Work out the finished part from the listing and answer in its coordinate system (mm). Face numbers are marked on the shaded views. A direction names the side the tool comes from. Coordinates: 2 decimals unless noted, no trailing zeros. Order: outer loops, then holes, each group sorted by start corner. A loop starts at its lowest first (then second) coordinate and runs counter-clockwise, first axis right, second up. Notation, with made-up numbers: M 11,-10.75 L 49,-10.75 A20 ccw 49,-6.75 Z; hole C 51,21 d5. An arc over 180 degrees is marked long. Use a Markdown table: item, result.
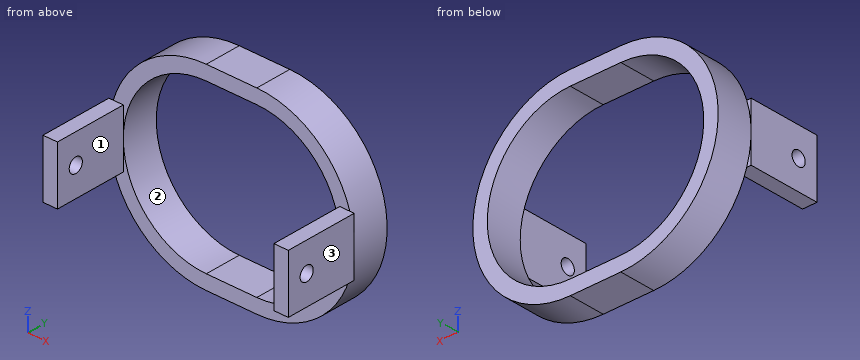
from build123d import *

# Parameters (mm, degrees)
EXTRUDE_1_DEPTH     = 10
SKETCH_3_W          = 4
SKETCH_3_H          = 16
EXTRUDE_2_DEPTH     = 20
SKETCH_5_R          = 2
CUT_EXTRUDE_2_DEPTH = 69


with BuildPart() as part:
    # 草图2 → 凸台-拉伸1 (new body)
    with BuildSketch(Plane(origin=(0, 0, 0), x_dir=(1, 0, 0), z_dir=(0, 1, 0))):
        with BuildLine():
            Line((-7, 27), (7, 27))
            ThreePointArc((7, 27), (34, 0), (7, -27))
            Line((7, -27), (-7, -27))
            ThreePointArc((-7, -27), (-34, 0), (-7, 27))
        make_face()
        with BuildLine():
            Line((-7, 23), (7, 23))
            ThreePointArc((7, 23), (30, 0), (7, -23))
            Line((7, -23), (-7, -23))
            ThreePointArc((-7, -23), (-30, 0), (-7, 23))
        make_face(mode=Mode.SUBTRACT)
    extrude(amount=EXTRUDE_1_DEPTH)

    # 草图3 → 凸台-拉伸2 (add)
    with BuildSketch(Plane.XZ):
        with Locations((-32, 0)):
            Rectangle(SKETCH_3_W, SKETCH_3_H)
        with Locations((32, 0)):
            Rectangle(SKETCH_3_W, SKETCH_3_H)
    extrude(amount=EXTRUDE_2_DEPTH)

    # 草图5 → 切除-拉伸2 (cut, through all)
    with BuildSketch(Plane(origin=(34, 0, 0), x_dir=(0, 0, -1), z_dir=(1, 0, 0))):
        with Locations((0, -14.426533044)):
            Circle(SKETCH_5_R)
    extrude(amount=-CUT_EXTRUDE_2_DEPTH, mode=Mode.SUBTRACT)


solid = part.part
(1) Given P1, Ø1.2, axis at x = 31, y = -14, coming from the +Z side; P2, Ø1.2, axis at x = -31.5, y = -7, coming from the -Z side; P3, Ø12, axis at x = -25, y = 6.5, coming from the -Z side, each flat-ended and moving along its own axis, determine where each tip first touches the part or whether it passes through.
Conclusion:
| item | result |
|---|---|
| P1 | z = 8 |
| P2 | z = -8 |
| P3 | z = -24.19 |
(2) A cutting plane is placed at C-C (x = 14). Determine the outline of the cut face in (y, z).
Conclusion:
| item | result |
|---|---|
| outline | M 0,-26.08 L 10,-26.08 L 10,-21.91 L 0,-21.91 Z; M 0,21.91 L 10,21.91 L 10,26.08 L 0,26.08 Z |
(3) Straight lines are drawn through the part: L1, parallel to Z at x = -4.5, y = 8.5; L2, parallel to Y at x = -32.85, z = 0; L3, parallel to X at y = -17.5, z = -3. For each, find the intervals that lie inside material, in ascending order.
Conclusion:
| item | result |
|---|---|
| L1 | -27 to -23, 23 to 27 |
| L2 | -20 to -16.43, -12.43 to 10 |
| L3 | -34 to -30, 30 to 34 |
(4) A cutting plane is placed at A-A (z = 4). Determine the outline of the cut face in (x, y), then the cut area to 3 significant figures.
Conclusion:
| item | result |
|---|---|
| outline | M -34,-20 L -30,-20 L -30,0 L -29.65,0 L -29.65,10 L -33.7,10 L -33.7,0 L -34,0 Z; M 29.65,0 L 30,0 L 30,-20 L 34,-20 L 34,0 L 33.7,0 L 33.7,10 L 29.65,10 Z |
| area | 241 mm2 |
(5) A cutting plane is placed at D-D (y = 1.25). Determine the outline of the cut face in (x, z), then the cut area to 3 significant figures.
Conclusion:
| item | result |
|---|---|
| outline | M -7,-27 L 7,-27 A27 ccw 7,27 L -7,27 A27 ccw Z; hole M -7,-23 L 7,-23 A23 ccw 7,23 L -7,23 A23 ccw Z |
| area | 740 mm2 |
(6) A cutting plane is placed at B-B (y = -6.25). Determine the outline of the cut face in (x, z), then the cut area to 3 significant figures.
Conclusion:
| item | result |
|---|---|
| outline | M -34,-8 L -30,-8 L -30,8 L -34,8 Z; M 30,-8 L 34,-8 L 34,8 L 30,8 Z |
| area | 128 mm2 |
(7) Which of the six approach directions +Z, -Z, +X, -X, +Y, -Y give full straight-line access (tool end or side, diameter ignored) to the marked faces 1, 2 and 3?
Conclusion:
| item | result |
|---|---|
| face 1 | +Z, -Z, -Y |
| face 2 | +Y, -Y |
| face 3 | +Z, -Z, +X, +Y, -Y |
